from build123d import *

# Parameters (mm, degrees)
EXTRUDE_1_DEPTH     = 26
SKETCH_2_R          = 3.5
SKETCH_2_R_2        = 4.5
CUT_EXTRUDE_1_DEPTH = 26
SKETCH_2_3_R        = 7.5
SKETCH_2_3_R_2      = 4.5
CUT_EXTRUDE_2_DEPTH = 5


with BuildPart() as part:
    # Sketch 1 → Extrude 1 (new body)
    with BuildSketch(Plane.XY):
        Polygon((0, 0), (40, 0), (40, 9), (39, 10), (9.862873216, 10), (7.811286052, 8.025146032), (6.29823885, 9.580536944), (7.811286052, 11.052393193), (7.811286052, 21.063841402), (6.900613284, 22), (1.900613284, 22), (0, 10), align=None)
    extrude(amount=EXTRUDE_1_DEPTH)

    # Sketch 2 → Cut-Extrude 1 (cut)
    with BuildSketch(Plane(origin=(0, 10, 0), x_dir=(1, 0, 0), z_dir=(0, 1, 0))):
        with Locations(Location((14.862873216, -21, 0), (0, 0, 270))):
            Circle(SKETCH_2_R)
        with Locations(Location((24.431436608, -13, 0), (0, 0, 270))):
            Circle(SKETCH_2_R_2)
        with Locations(Location((34, -5, 0), (0, 0, 270))):
            Circle(SKETCH_2_R)
    extrude(amount=-CUT_EXTRUDE_1_DEPTH, mode=Mode.SUBTRACT)

    # Sketch 2_3 → Cut-Extrude 2 (cut)
    with BuildSketch(Plane(origin=(0, 10, 0), x_dir=(1, 0, 0), z_dir=(0, 1, 0))):
        with Locations(Location((24.431436608, -13, 0), (0, 0, 270))):
            Circle(SKETCH_2_3_R)
        with Locations(Location((24.431436608, -13, 0), (0, 0, 270))):
            Circle(SKETCH_2_3_R_2, mode=Mode.SUBTRACT)
    extrude(amount=-CUT_EXTRUDE_2_DEPTH, mode=Mode.SUBTRACT)


solid = part.part
Can you work these out from the model? Positions are in its coordinate system, mm. A direction names the side the tool comes from. Coordinates: 2 decimals unless noted, no trailing zeros. Loops run counter-clockwise (first coordinate to the right, second up) from the corner with the lowest first, then second, coordinate; pieces in that order, holes last. Notation, with made-up numbers: (-21.5, 65.5) - (-17.5, 65.5) arc R19 ccw to (-17.5, 81.5) - close; hole circle Ø1 at (-12.75, -10.75). An arc over 180 degrees is marked (long way). Answer as a JSON object with one key per item and string values. Group by question number.
Item 1: If we section it at C-C (y = 1.5): List the corners of the cut face in (x, z) for me, plus the area to 3 significant figures.
Item 2: If we mould it in two halves opening along Z, with no side actions, what happens to faces 4 (the face through (15, 6, 26)), 5 (the face through (19.7, 0, 12.8)), 6 (the face through (15, 6, 0)), 7 (the face through (37.47, 5.07, 4.54))? For each: released by +Z, released by -Z, zero draft, split by the parting line, or undercut.
Item 3: If we section it at B-B (x = 34): List the corners of the cut face in (y, z) for me.
Item 4: For pin 1 (8 mm diameter, centred on x = 27, z = 8.5, fed in from +Y); pin 2 (3 mm diameter, centred on y = 14, z = 9.5, fed in from +X); pin 3 (4.5 mm diameter, centred on x = 27.5, z = 12, fed in from +Y), each with a flat end and sliding along its axis, tell me the tip position at first contact or that it passes through.
Item 5: On a 3-axis mill with a long thin cutter (end or side, diameter ignored), from which of +Z, -Z, +X, -X, +Y, -Y can I reach the whole of each face in a straight line? I mean faces 1 (the face through (19.5, 5, 12.9)), 2 (the face through (7.07, 8.79, 12.82)), 3 (the face through (25, 10, 4)). Say none if no direction works.
Item 6: If I drill on L1, parallel to X at y = 1.4, z = 13; L2, parallel to X at y = 8.75, z = 6.5; L3, parallel to X at y = 6, z = 5, over which ranges is the centre line in solid material (lowest first)? Write a range as from..to.
Item 7: If we section it at A-A (z = 13): List the corners of the cut face in (x, y) for me, plus the area to 3 significant figures.
Item 8: If we section it at D-D (z = 5): List the corners of the cut face in (x, y) for me, plus the area to 3 significant figures.
Returned:
{
 "1": {"outline": "(0, 0) - (40, 0) - (40, 26) - (0, 26) - close; hole circle Ø7 at (14.86, 21); hole circle Ø9 at (24.43, 13); hole circle Ø7 at (34, 5)", "area": "899 mm²"},
 "2": {"face 4": "released by +Z", "face 5": "zero draft", "face 6": "released by -Z", "face 7": "undercut"},
 "3": {"outline": "(0, 0) - (10, 0) - (10, 1.5) - (0, 1.5) - close; (0, 8.5) - (10, 8.5) - (10, 26) - (0, 26) - close"},
 "4": {"pin 1": "stops at y = 10", "pin 2": "stops at x = 7.81", "pin 3": "stops at y = 5"},
 "5": {"face 1": "+Y", "face 2": "+Z, -Z", "face 3": "+Z, -Z, +X, +Y"},
 "6": {"L1": "x = 0..19.93, 28.93..40", "L2": "x = 0..7.11, 8.56..20.69, 28.17..30.84, 37.16..40", "L3": "x = 0..30.5, 37.5..40"},
 "7": {"outline": "(0, 0) - (19.93, 0) - (19.93, 5) - (16.93, 5) - (16.93, 10) - (9.86, 10) - (7.81, 8.03) - (6.3, 9.58) - (7.81, 11.05) - (7.81, 21.06) - (6.9, 22) - (1.9, 22) - (0, 10) - close; (28.93, 0) - (40, 0) - (40, 9) - (39, 10) - (31.93, 10) - (31.93, 5) - (28.93, 5) - close", "area": "357 mm²"},
 "8": {"outline": "(0, 0) - (30.5, 0) - (30.5, 10) - (9.86, 10) - (7.81, 8.03) - (6.3, 9.58) - (7.81, 11.05) - (7.81, 21.06) - (6.9, 22) - (1.9, 22) - (0, 10) - close; (37.5, 0) - (40, 0) - (40, 9) - (39, 10) - (37.5, 10) - close", "area": "407 mm²"}
}
